```python
from build123d import *

# Parameters (mm, degrees)
SKETCH1_R           = 18.0975
SKETCH1_R_2         = 1.4605
SKETCH1_W           = 3.175
SKETCH1_H           = 6
BOSS_EXTRUDE1_DEPTH = 3.175


with BuildPart() as part:
    # Sketch1 → Boss-Extrude1 (new body)
    with BuildSketch(Plane(origin=(0, 0, 0), x_dir=(1, 0, 0), z_dir=(0, 1, 0))):
        with Locations(Location((0, 0, 0), (0, 0, 270))):
            Circle(SKETCH1_R)
        with Locations(Location((0, 0, 0), (0, 0, 270))):
            Circle(SKETCH1_R_2, mode=Mode.SUBTRACT)
        Polygon((1.5875, -4), (1.5875, -3), (-1.5875, -3), (-1.5875, -11), (1.5875, -11), (1.5875, -10), (4.7625, -10), (4.7625, -4), align=None, mode=Mode.SUBTRACT)
        with Locations((3.175, 7)):
            Rectangle(SKETCH1_W, SKETCH1_H, mode=Mode.SUBTRACT)
    extrude(amount=BOSS_EXTRUDE1_DEPTH)


solid = part.part
```
Verification items for the finished model (mm, model axes). A direction names the side the tool comes from. Give positions to 0.01 mm unless a question says otherwise; leave off trailing zeros. Order: outer loops, then holes, each group sorted by start corner. A loop starts at its lowest first (then second) coordinate and runs counter-clockwise, first axis right, second up. Notation, with made-up numbers: (59.25, -12) - (70.25, -12) arc R16 cw to (70.25, 17) - close; hole circle Ø6 at (83.25, 17.25). An arc over 180 degrees is marked (long way). Answer as CSV lines item,"result". Start each with the question number.
Item 1: Access from +Z, -Z, +X, -X, +Y, -Y to the whole of each face (thin tool, end or side, straight path). Record for faces 1 (the face through (3, 2, 10)), 2 (the face through (-4, 3.175, 0)).
Item 2: Material ranges on L1, parallel to X at y = 2.2, z = 0; L2, parallel to Z at x = -0.5, y = 2.45; L3, parallel to Z at x = 4, y = 1.25, recorded low to high.
Item 3: Section check B-B, the plane y = 0.95. Record the boundary of the cut face in (x, z) (1 decimal), plus the area to 3 significant figures.
Item 4: Gauge pin test, flat ends, axial feed: pin 1 (1.6 mm diameter, centred on y = 2, z = -6, fed in from -X); pin 2 (1 mm diameter, centred on x = 3.5, y = 1.5, fed in from +Z); pin 3 (3 mm diameter, centred on x = -3.5, z = 6.5, fed in from -Y); pin 4 (0.8 mm diameter, centred on y = 1, z = 10.5, fed in from -X). Record the tip position at first contact, or that the pin passes through.
Item 5: Section check A-A, the plane z = 0. Record the boundary of the cut face in (x, y) (1 decimal), plus the area to 3 significant figures.
Item 6: Section check C-C, the plane x = 0. Record the boundary of the cut face in (y, z) (1 decimal).
Item 7: Mould release check, pull along Z, two halves, no side actions. Record for faces 3 (the face through (17.943, 1.565, -2.356)), 4 (the face through (-4, 0, 0)), 5 (the face through (1.588, 2, -7)): released by +Z, released by -Z, zero draft, split by the parting line, or undercut.
Item 8: Section check D-D, the plane x = -7.5. Record the boundary of the cut face in (y, z) (3 decimals).
Filled in:
1,face 1,"+Y, -Y"
1,face 2,"+Z, -Z, +X, -X, +Y"
2,L1,"-18.1 to -1.46, 1.46 to 18.1"
2,L2,"-18.09 to -1.37, 1.37 to 3, 11 to 18.09"
2,L3,"-17.65 to -10, -4 to 4, 10 to 17.65"
3,outline,"circle Ø36.2 at (0, 0); hole (-1.6, 3) - (1.6, 3) - (1.6, 4) - (4.8, 4) - (4.8, 10) - (1.6, 10) - (1.6, 11) - (-1.6, 11) - close; hole circle Ø2.9 at (0, 0); hole (1.6, -10) - (4.8, -10) - (4.8, -4) - (1.6, -4) - close"
3,area,"959 mm^2"
4,pin 1,"x = -17.33"
4,pin 2,"z = 17.85"
4,pin 3,"y = 0"
4,pin 4,"x = -15.02"
5,outline,"(-18.1, 0) - (-1.5, 0) - (-1.5, 3.2) - (-18.1, 3.2) - close; (1.5, 0) - (18.1, 0) - (18.1, 3.2) - (1.5, 3.2) - close"
5,area,"106 mm^2"
6,outline,"(0, -18.1) - (3.2, -18.1) - (3.2, -1.5) - (0, -1.5) - close; (0, 1.5) - (3.2, 1.5) - (3.2, 3) - (0, 3) - close; (0, 11) - (3.2, 11) - (3.2, 18.1) - (0, 18.1) - close"
7,face 3,"split by the parting line"
7,face 4,"zero draft"
7,face 5,"undercut"
8,outline,"(0, -16.47) - (3.175, -16.47) - (3.175, 16.47) - (0, 16.47) - close"
